Input: part model. Units: mm. Frame: model coordinates. A direction names the side the tool comes from. Give positions to 0.01 mm unless a question says otherwise; leave off trailing zeros. Loops run counter-clockwise (first coordinate to the right, second up) from the corner with the lowest first, then second, coordinate; pieces in that order, holes last. Notation, with made-up numbers: (67, 37) - (87, 37) arc R5 ccw to (87, 45) - close; hole circle Ø6 at (62, 15.25). An arc over 180 degrees is marked (long way). Answer as a JSON object with one key per item and string values. Group by question number.
(1) Access query for faces 5 (the flat face through (-50.8, 0, 9)), 6 (the flat face through (-1, 26, 12.7)). Directions: +Z, -Z, +X, -X, +Y, -Y. A direction counts if a zero-diameter tool reaches every point of the face in a straight line with its end or side. Return the directions, or none.
(2) Mould query, pull axis Y, two halves, no side actions, for faces 1 (the flat face through (50.8, 0, 3)), 2 (the flat face through (1, -25.4, 9)), 3 (the flat face through (0, 26.988, 6)), 4 (the flat face through (-2, -26.988, 6)). Classes: +Y half, -Y half, draft (parallel to the pull), parting line (faces both ways), or undercut.
(3) Pin query (flat end, axial travel): P1, Ø13.5, axis at x = 3, y = -0.5, coming from the +Z side; P2, Ø0.5, axis at y = -24.5, z = 9, coming from the +X side. Return the tip coordinate at first contact, or that it passes through.
(4) Material intervals for L1, parallel to Y at x = -34.5, z = 7 (1 decimal); L2, parallel to Z at x = -6, y = -18.5; L3, parallel to X at y = 0, z = 11.75, sorted ascending.
(5) Section query B-B (y = -8). Return loops of the section in (x, z), plus the area to 3 significant figures.
```python
from build123d import *

# Parameters (mm, degrees)
F0_W     = 101.6
F0_H     = 50.8
F1_DEPTH = 6.35
F3_DEPTH = 12.7


with BuildPart() as f1:
    # F0 (on Top) → F1 (new body)
    with BuildSketch(Plane.XY):
        Rectangle(F0_W, F0_H)
    extrude(amount=F1_DEPTH)

    # F2 (on Top) → F3 (join)
    with BuildSketch(Plane.XY):
        Polygon((50.8, 25.4), (50.8, 26.9875), (-52.3875, 26.9875), (-52.3875, -26.9875), (50.8, -26.9875), (50.8, -25.4), (-50.8, -25.4), (-50.8, -23.8125), (50.8, -23.8125), (50.8, -22.225), (-50.8, -22.225), (-50.8, 22.225), (50.8, 22.225), (50.8, 23.8125), (-50.8, 23.8125), (-50.8, 25.4), align=None)
    extrude(amount=F3_DEPTH)


solid = f1.part
```
Recorded:
{
 "1": {"face 5": "+Z, +X", "face 6": "+Z, +X, -X, +Y, -Y"},
 "2": {"face 1": "draft", "face 2": "undercut", "face 3": "+Y half", "face 4": "-Y half"},
 "3": {"P1": "stops at z = 6.35", "P2": "stops at x = -50.8"},
 "4": {"L1": "y = -27 to -25.4, -23.8 to -22.2, 22.2 to 23.8, 25.4 to 27", "L2": "z = 0 to 6.35", "L3": "x = -52.39 to -50.8"},
 "5": {"outline": "(-52.39, 0) - (50.8, 0) - (50.8, 6.35) - (-50.8, 6.35) - (-50.8, 12.7) - (-52.39, 12.7) - close", "area": "665 mm^2"}
}
